Here's how the part is built. I have some questions about the finished solid (model axes, mm). Face numbers are marked on the shaded views. A direction names the side the tool comes from. Give positions to 0.01 mm unless a question says otherwise; leave off trailing zeros. Loops run counter-clockwise (first coordinate to the right, second up) from the corner with the lowest first, then second, coordinate; pieces in that order, holes last.
Q1. If we section it at B-B (z = 5.5): Please give me the cut outline in (x, y), plus the area to 3 significant figures.
Q2. We'd pull the mould along Z, two halves only. Please class the marked faces 1, 2 and 3: +Z half, -Z half, draft (parallel to the pull), parting line (faces both ways), or undercut.
Q3. If we section it at C-C (x = 5.5): Please give me the cut outline in (y, z).
Q4. If we section it at A-A (z = 17.75): Please give me the cut outline in (x, y) (3 decimals).
Q5. For the marked faces 4 and 5, which set-ups out of +Z, -Z, +X, -X, +Y, -Y let a thin tool reach every point of the face, with its end or its side?
Q6. Will these pins go through, and if not, where does the flat tip stop? P1, Ø1.5, axis at x = 4, z = 2, coming from the +Y side; P2, Ø8, axis at x = -12, z = 22.5, coming from the -Y side; P3, Ø4, axis at y = 1.5, z = 18.5, coming from the +X side.
Q7. I need wall thicknesses on line 1 (X direction, y = 4.5, z = 32.5) (3 decimals); line 2 (X direction, y = 1, z = 14.5); line 3 (Z direction, x = 12.15, y = 0) (3 decimals). Which ranges of each line are inside material? Lowest first, please.
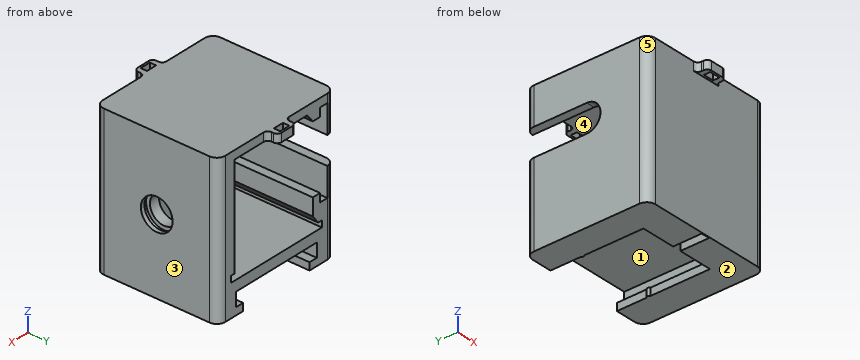
from build123d import *

# Parameters (mm, degrees)
SKETCH1_W                = 32
SKETCH1_H                = 29
BOSS_EXTRUDE1_DEPTH      = 35
FILLET1_R                = 2
SLOT_FOR_COIL_DEPTH      = 1
SLOT_FOR_COIL_DEPTH_BACK = 30
BOSS_EXTRUDE2_DEPTH      = 7
BOSS_EXTRUDE3_DEPTH      = 1.75
SKETCH5_W                = 2
SKETCH5_H                = 7
CUT_EXTRUDE2_DEPTH       = 33
CUT_EXTRUDE3_DEPTH       = 22
SKETCH7_W                = 2
SKETCH7_H                = 33
BOSS_EXTRUDE4_DEPTH      = 0.25
FILLET2_R                = 6
CUT_EXTRUDE5_DEPTH       = 4.5
SKETCH14_W               = 2.5
SKETCH14_H               = 20
CUT_EXTRUDE6_DEPTH       = 22
SKETCH16_W               = 2
SKETCH16_H               = 4
SKETCH16_H_2             = 2
BOSS_EXTRUDE5_DEPTH      = 22
BOSS_EXTRUDE6_DEPTH      = 22
SKETCH21_W               = 5
SKETCH21_H               = 2
BOSS_EXTRUDE7_DEPTH      = 2.5
SKETCH23_W               = 2.5
SKETCH23_H               = 1.5
CUT_EXTRUDE7_DEPTH       = 2
FILLET3_R                = 1


with BuildPart() as part:
    # Sketch1 → Boss-Extrude1 (new body)
    with BuildSketch(Plane.XY):
        Rectangle(SKETCH1_W, SKETCH1_H)
    extrude(amount=BOSS_EXTRUDE1_DEPTH)

    # Fillet1
    fillet1_edges = [part.edges().sort_by_distance(p)[0] for p in [
        (16, -14.5, 17.5),
        (-16, -14.5, 17.5),
        (-16, 14.5, 17.5),
        (16, 14.5, 17.5),
    ]]
    fillet(fillet1_edges, radius=FILLET1_R)

    # Sketch2 → Slot for Coil (cut, two sides)
    with BuildSketch(Plane.XZ.offset(14.5)) as slot_for_coil_sk:
        Polygon((-9.125, 0), (-9.125, 1.75), (-11.125, 1.75), (-11.125, 5), (11.125, 5), (11.125, 1.75), (9.125, 1.75), (9.125, 0), align=None)
    extrude(amount=SLOT_FOR_COIL_DEPTH, mode=Mode.SUBTRACT)
    extrude(slot_for_coil_sk.sketch, amount=-SLOT_FOR_COIL_DEPTH_BACK, mode=Mode.SUBTRACT)

    # Sketch3 → Boss-Extrude2 (add)
    with BuildSketch(Plane.XZ.offset(14.5)):
        Polygon((-9.125, 0), (-9.125, 1.75), (-11.125, 1.75), (-11.125, 5), (11.125, 5), (11.125, 1.75), (9.125, 1.75), (9.125, 0), align=None)
    extrude(amount=-BOSS_EXTRUDE2_DEPTH)

    # Sketch4 → Boss-Extrude3 (add)
    with BuildSketch(Plane(origin=(0, 0, 1.75), x_dir=(-1, 0, 0), z_dir=(0, 0, -1))):
        with BuildLine():
            Line((-9.125, 7.5), (-9.125, 6.5))
            ThreePointArc((-9.125, 6.5), (-8.875, 7), (-9.125, 7.5))
        make_face()
    boss_extrude3 = extrude(amount=BOSS_EXTRUDE3_DEPTH)

    # Mirror1: Boss-Extrude3 across plane
    add(boss_extrude3.mirror(Plane(origin=(0, 0, 0), x_dir=(0, 0, 1), z_dir=(1, 0, 0))))

    # Sketch5 → Cut-Extrude2 (cut)
    with BuildSketch(Plane(origin=(0, 0, 0), x_dir=(-1, 0, 0), z_dir=(0, 0, -1))):
        with Locations((0, -11)):
            Rectangle(SKETCH5_W, SKETCH5_H)
    extrude(amount=-CUT_EXTRUDE2_DEPTH, mode=Mode.SUBTRACT)

    # Sketch6 → Cut-Extrude3 (cut)
    with BuildSketch(Plane(origin=(0, 14.5, 0), x_dir=(1, 0, 0), z_dir=(0, 1, 0))):
        Polygon((-12.5, -7.5), (-12.5, -9), (-11.5, -9), (-11.5, -33), (11.5, -33), (11.5, -9), (12.5, -9), (12.5, -7.5), align=None)
    extrude(amount=-CUT_EXTRUDE3_DEPTH, mode=Mode.SUBTRACT)

    # Sketch7 → Boss-Extrude4 (add)
    with BuildSketch(Plane.XZ.offset(14.5)):
        with Locations((0, 16.5)):
            Rectangle(SKETCH7_W, SKETCH7_H)
    extrude(amount=-BOSS_EXTRUDE4_DEPTH)

    # Fillet2
    fillet2_edges = [part.edges().sort_by_distance(p)[0] for p in [
        (0, -14.25, 33),
    ]]
    fillet(fillet2_edges, radius=FILLET2_R)

    # Sketch9 → Cut-Revolve1 (revolve, cut)
    with BuildSketch(Plane(origin=(0, 0, 17.75), x_dir=(-1, 0, 0), z_dir=(0, 0, -1))):
        Polygon((-15, 4.25), (-14, 4.25), (-14, 3.325), (-11.5, 3.325), (-11.5, 0), (-16, 0), (-16, 3.75), (-15, 3.75), align=None)
    revolve(axis=Axis((16, 0, 17.75), (-1, 0, 0)), mode=Mode.SUBTRACT)

    # Sketch11 → Cut-Extrude5 (cut)
    with BuildSketch(Plane(origin=(-16, 0, 44), x_dir=(0, 0, -1), z_dir=(1, 0, 0))):
        with BuildLine():
            Line((24.25, 25), (24.25, 0))
            ThreePointArc((24.25, 0), (21, -3.25), (17.75, 0))
            Line((17.75, 0), (17.75, 25))
            ThreePointArc((17.75, 25), (21, 28.25), (24.25, 25))
        make_face()
    extrude(amount=CUT_EXTRUDE5_DEPTH, mode=Mode.SUBTRACT)

    # Sketch14 → Cut-Extrude6 (cut)
    with BuildSketch(Plane(origin=(0, 14.5, 0), x_dir=(1, 0, 0), z_dir=(0, 1, 0))):
        with Locations((-12.75, -23)):
            Rectangle(SKETCH14_W, SKETCH14_H)
    extrude(amount=-CUT_EXTRUDE6_DEPTH, mode=Mode.SUBTRACT)

    # Sketch16 → Boss-Extrude5 (add)
    with BuildSketch(Plane(origin=(0, 14.5, 0), x_dir=(1, 0, 0), z_dir=(0, 1, 0))):
        with Locations((-11, -13)):
            Rectangle(SKETCH16_W, SKETCH16_H)
        with Locations((-11, -32)):
            Rectangle(SKETCH16_W, SKETCH16_H_2)
    extrude(amount=-BOSS_EXTRUDE5_DEPTH)

    # Sketch20 → Boss-Extrude6 (add)
    with BuildSketch(Plane(origin=(0, 14.5, 0), x_dir=(1, 0, 0), z_dir=(0, 1, 0))):
        Polygon((-11.5, -9), (-10, -11), (-11.5, -11), align=None)
        Polygon((-10, -31), (-8.5, -33), (-10, -33), align=None)
    extrude(amount=-BOSS_EXTRUDE6_DEPTH)

    # Sketch21 → Boss-Extrude7 (add)
    with BuildSketch(Plane(origin=(0, 14.5, 0), x_dir=(-1, 0, 0), z_dir=(0, 1, 0))):
        with Locations((0, 34)):
            Rectangle(SKETCH21_W, SKETCH21_H)
    boss_extrude7 = extrude(amount=BOSS_EXTRUDE7_DEPTH)

    # Sketch23 → Cut-Extrude7 (cut)
    with BuildSketch(Plane.XY.offset(35)):
        with Locations((0, 15.75)):
            Rectangle(SKETCH23_W, SKETCH23_H)
    cut_extrude7 = extrude(amount=-CUT_EXTRUDE7_DEPTH, mode=Mode.SUBTRACT)

    # Mirror3: Boss-Extrude7, Cut-Extrude7 across plane
    add(boss_extrude7.mirror(Plane.ZX))
    add(cut_extrude7.mirror(Plane.ZX), mode=Mode.SUBTRACT)

    # Fillet3
    fillet3_edges = [part.edges().sort_by_distance(p)[0] for p in [
        (2.5, 14.5, 34),
        (-2.5, 14.5, 34),
        (2.5, 17, 34),
        (-2.5, 17, 34),
        (2.5, -17, 34),
        (-2.5, -17, 34),
        (2.5, -14.5, 34),
        (-2.5, -14.5, 34),
    ]]
    fillet(fillet3_edges, radius=FILLET3_R)


solid = part.part
Check sheet entries:
1. outline: (-16, -12.5) arc R2 ccw to (-14, -14.5) - (14, -14.5) arc R2 ccw to (16, -12.5) - (16, 12.5) arc R2 ccw to (14, 14.5) - (-14, 14.5) arc R2 ccw to (-16, 12.5) - close; hole (-1, -14.25) - (1, -14.25) - (1, -7.5) - (-1, -7.5) - close
1. area: 911 mm2
2. face 1: undercut
2. face 2: -Z half
2. face 3: draft
3. outline: (-14.5, 0) - (-7.5, 0) - (-7.5, 5) - (14.5, 5) - (14.5, 7.5) - (-7.5, 7.5) - (-7.5, 33) - (14.5, 33) - (14.5, 35) - (-14.5, 35) - close
4. outline: (-16, -12.5) arc R2 ccw to (-14, -14.5) - (14, -14.5) arc R2 ccw to (16, -12.5) - (16, -3.75) - (15, -3.75) - (15, -4.25) - (14, -4.25) - (14, -3.325) - (11.5, -3.325) - (11.5, -7.5) - (1, -7.5) - (1, -14.25) - (-1, -14.25) - (-1, -7.5) - (-14, -7.5) - (-14, 14.5) arc R2 ccw to (-16, 12.5) - close; (11.5, 3.325) - (14, 3.325) - (14, 4.25) - (15, 4.25) - (15, 3.75) - (16, 3.75) - (16, 12.5) arc R2 ccw to (14, 14.5) - (11.5, 14.5) - close
5. face 4: +Y
5. face 5: +Z, -Z, -X, -Y
6. P1: stops at y = -7.5
6. P2: stops at y = -14.5
6. P3: stops at x = 14
7. line 1: x = -16 to -14, -12 to -8.875, 11.5 to 16
7. line 2: x = -16 to -14, -12 to -10, 11.5 to 14
7. line 3: z = 0 to 7.5, 9 to 14.425, 21.075 to 35
